Check sheet for the modelled part. Datum: model origin and axes. Units: mm. Face numbers are marked on the shaded views. A direction names the side the tool comes from. Round coordinates to 2 decimals unless told otherwise and drop trailing zeros. Order: outer loops, then holes, each group sorted by start corner. A loop starts at its lowest first (then second) coordinate and runs counter-clockwise, first axis right, second up. Notation, with made-up numbers: (-25, -21.5) -> (18, -21.5) arc R17 cw to (18, 8.5) -> close; hole circle Ø4 at (41.25, 5.5). An arc over 180 degrees is marked (long way). Answer in a Markdown table with one row per item. Add a question column.
1. Sectioned sample at C-C, the plane z = 6. Record the boundary of the cut face in (x, y), then the cut area to 3 significant figures.
2. Depth check by flat-ended pin: P1, Ø1, axis at x = -24, z = 12.5, coming from the -Y side. Enter the tip coordinate at first touch or a pass-through.
3. Material ranges on L1, parallel to Z at x = -54.5, y = -22; L2, parallel to X at y = -21, z = -28; L3, parallel to Z at x = -27, y = -18, recorded low to high. Write a range as from..to.
4. Draft check along X on the marked faces 1, 2 and 3. Enter one of: +X half, -X half, draft (parallel to the pull), parting line (faces both ways), or undercut.
5. Access from +Z, -Z, +X, -X, +Y, -Y to the whole of each face (thin tool, end or side, straight path). Record for the marked faces 4 and 5.
6. Sectioned sample at A-A, the plane y = -25.5. Record the boundary of the cut face in (x, z).
7. Sectioned sample at B-B, the plane x = 6.5. Record the boundary of the cut face in (y, z).
```python
from build123d import *

# Parameters (mm, degrees)
F0_W     = 101.6
F0_H     = 76.2
F0_W_2   = 86.36
F0_H_2   = 60.96
F1_DEPTH = 38.1
F2_DEPTH = 12.7
F3_W     = 25.4
F3_H     = 7.263597
F4_DEPTH = 25.4
F5_W     = 25.4
F5_H     = 7.33001
F6_DEPTH = 25.4


with BuildPart() as f1:
    # F0 (on Front) → F1 (new body)
    with BuildSketch(Plane.XZ):
        with Locations((-18.985149, -0.786755)):
            Rectangle(F0_W, F0_H)
        with Locations((-18.985149, -0.786755)):
            Rectangle(F0_W_2, F0_H_2, mode=Mode.SUBTRACT)
    extrude(amount=F1_DEPTH)

    # F0 (on Front) → F2 (join)
    with BuildSketch(Plane.XZ):
        with Locations((-18.985149, -0.786755)):
            Rectangle(F0_W_2, F0_H_2)
    extrude(amount=F2_DEPTH)

    # F3 (on face) → F4 (join)
    with BuildSketch(Plane.YZ.offset(-62.165149)):
        with Locations((-25.4, 21.148253)):
            Rectangle(F3_W, F3_H)
    extrude(amount=F4_DEPTH)

    # F5 (on face) → F6 (join)
    with BuildSketch(Plane.YZ.offset(-62.165149)):
        with Locations((-25.4, 8.285583)):
            Rectangle(F5_W, F5_H)
    extrude(amount=F6_DEPTH)


solid = f1.part
```
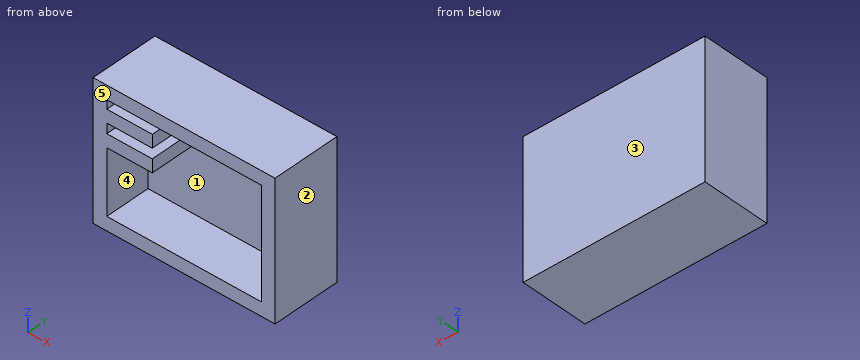
Answer key:
| question | item | result |
|---|---|---|
| 1 | outline | (-69.79, -38.1) -> (-36.77, -38.1) -> (-36.77, -12.7) -> (24.19, -12.7) -> (24.19, -38.1) -> (31.81, -38.1) -> (31.81, 0) -> (-69.79, 0) -> close |
| 1 | area | 2,320 mm² |
| 2 | P1 | stops at y = -12.7 |
| 3 | L1 | z = -38.89..-31.27, 4.62..11.95, 17.52..24.78, 29.69..37.31 |
| 3 | L2 | x = -69.79..-62.17, 24.19..31.81 |
| 3 | L3 | z = -38.89..-31.27, 29.69..37.31 |
| 4 | face 1 | undercut |
| 4 | face 2 | +X half |
| 4 | face 3 | draft |
| 5 | face 4 | -Y |
| 5 | face 5 | +Z, -Z, +X, -X, -Y |
| 6 | outline | (-69.79, -38.89) -> (31.81, -38.89) -> (31.81, 37.31) -> (-69.79, 37.31) -> close; hole (-62.17, -31.27) -> (24.19, -31.27) -> (24.19, 29.69) -> (-62.17, 29.69) -> (-62.17, 24.78) -> (-36.77, 24.78) -> (-36.77, 17.52) -> (-62.17, 17.52) -> (-62.17, 11.95) -> (-36.77, 11.95) -> (-36.77, 4.62) -> (-62.17, 4.62) -> close |
| 7 | outline | (-38.1, -38.89) -> (0, -38.89) -> (0, 37.31) -> (-38.1, 37.31) -> (-38.1, 29.69) -> (-12.7, 29.69) -> (-12.7, -31.27) -> (-38.1, -31.27) -> close |
